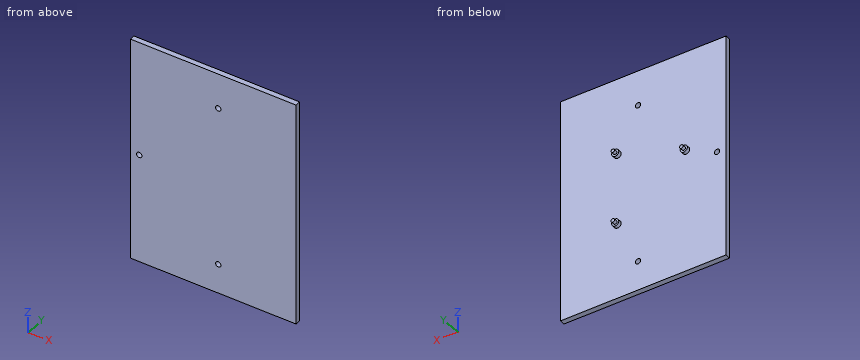
from build123d import *

# Parameters (mm, degrees)
SKETCH1_W           = 93.25
SKETCH1_H           = 125
BOSS_EXTRUDE1_DEPTH = 3
SKETCH3_R           = 1.5
CUT_EXTRUDE1_DEPTH  = 3
SKETCH4_R           = 2
SKETCH4_R_2         = 1
BOSS_EXTRUDE2_DEPTH = 2
SKETCH6_R           = 1
BOSS_EXTRUDE3_DEPTH = 4


with BuildPart() as part:
    # Sketch1 → Boss-Extrude1 (new body)
    with BuildSketch(Plane(origin=(0, 0, 0), x_dir=(1, 0, 0), z_dir=(0, 1, 0))):
        with Locations((-6.857134593, 56.824464746)):
            Rectangle(SKETCH1_W, SKETCH1_H)
    extrude(amount=BOSS_EXTRUDE1_DEPTH)

    # Sketch3 → Cut-Extrude1 (cut)
    with BuildSketch(Plane(origin=(0, 3, 0), x_dir=(1, 0, 0), z_dir=(0, 1, 0))):
        with Locations(Location((-3.982134593, 102.947941071, 0), (0, 0, 270))):
            Circle(SKETCH3_R)
    cut_extrude1 = extrude(amount=-CUT_EXTRUDE1_DEPTH, mode=Mode.SUBTRACT)

    # Sketch-Pattern1: Cut-Extrude1 at 2 more places
    with Locations((0, 0, 89), (-44.5, 0, 44.5)):
        add(cut_extrude1, mode=Mode.SUBTRACT)

    # Sketch4 → Boss-Extrude2 (add)
    with BuildSketch(Plane(origin=(0, 3, 0), x_dir=(1, 0, 0), z_dir=(0, 1, 0))):
        with Locations(Location((-31.082134593, 50.747941071, 0), (0, 0, 270))):
            Circle(SKETCH4_R)
        with Locations(Location((-31.082134593, 50.747941071, 0), (0, 0, 270))):
            Circle(SKETCH4_R_2, mode=Mode.SUBTRACT)
    boss_extrude2 = extrude(amount=BOSS_EXTRUDE2_DEPTH)

    # Sketch6 → Boss-Extrude3 (add)
    with BuildSketch(Plane(origin=(0, 3, 0), x_dir=(1, 0, 0), z_dir=(0, 1, 0))):
        with Locations(Location((-31.082134593, 50.747941071, 0), (0, 0, 270))):
            Circle(SKETCH6_R)
    boss_extrude3 = extrude(amount=BOSS_EXTRUDE3_DEPTH)

    # Sketch-Pattern2: Boss-Extrude2, Boss-Extrude3 at 2 more places
    with Locations((38.6, 0, -26.6), (38.6, 0, 13.2)):
        add(boss_extrude2)
        add(boss_extrude3)


solid = part.part
Read the model definition and answer for the solid it produces. Units are mm, in the model's axes. Round coordinates to 2 decimals unless told otherwise and drop trailing zeros. Write each loop counter-clockwise with the first axis right and the second up, starting at its lowest first coordinate (ties: lowest second). Pieces come first, ordered by that corner, then holes. Notation, with made-up numbers: M 80.25,67 L 123.25,67 A18 cw 123.25,77 Z; hole C 67.5,-1.75 d8. An arc over 180 degrees is marked long. Use a Markdown table: item, result.
1) Flat-ended cylindrical pins translate along their axes: pin 1 (3 mm diameter, centred on x = -33.5, z = -14.5, fed in from +Y); pin 2 (4 mm diameter, centred on y = 3.5, z = -93.5, fed in from +X). Find the tip coordinate at first contact, or state that the pin passes through.
Answers follow:
| item | result |
|---|---|
| pin 1 | stops at y = 3 |
| pin 2 | stops at x = 39.77 |
2) Straight lines are drawn through the part: line 1 along Y through (x, z) = (6.5, -83.5); line 2 along X through (y, z) = (3.75, -50.5); line 3 along X through (y, z) = (2.25, -59). For each, find the intervals that lie inside material, in ascending order. Write a range as [from, to].
Answers follow:
| item | result |
|---|---|
| line 1 | y = [0, 3] |
| line 2 | x = [-33.07, -29.1] |
| line 3 | x = [-53.48, -49.88], [-47.09, 39.77] |
3) The part is cut by section B-B (z = -94). Write down the section's boundary in (x, y).
Answers follow:
| item | result |
|---|---|
| outline | M -53.48,0 L 39.77,0 L 39.77,3 L -53.48,3 Z |
4) The part is cut by section A-A (x = -36). Write down the section's boundary in (y, z).
Answers follow:
| item | result |
|---|---|
| outline | M 0,-119.32 L 3,-119.32 L 3,5.68 L 0,5.68 Z |
